from build123d import *

# Parameters (mm, degrees)
SKETCH1_R           = 2.4
BOSS_EXTRUDE1_DEPTH = 5
SKETCH2_R           = 2.4
CUT_EXTRUDE1_DEPTH  = 5
CUT_EXTRUDE2_DEPTH  = 1
SKETCH5_R           = 5
SKETCH5_R_2         = 1
BOSS_EXTRUDE2_DEPTH = 3
SKETCH6_R           = 2
CUT_EXTRUDE3_DEPTH  = 1


with BuildPart() as part:
    # Sketch1 → Boss-Extrude1 (new body)
    with BuildSketch(Plane(origin=(0, 0, 0), x_dir=(0.999757303, -0.022030336, 0), z_dir=(0, 0, 1))):
        with BuildLine():
            Line((-49.372163993, 87.590629426), (-29.904437649, 103.275259833))
            ThreePointArc((-29.904437649, 103.275259833), (-22.873966299, 102.518640646), (-23.630585486, 95.488169295))
            Line((-23.630585486, 95.488169295), (-43.09831183, 79.803538889))
            ThreePointArc((-43.09831183, 79.803538889), (-50.12878318, 80.560158076), (-49.372163993, 87.590629426))
        make_face()
        with Locations((-26.767511567, 99.381714564)):
            Circle(SKETCH1_R, mode=Mode.SUBTRACT)
    extrude(amount=BOSS_EXTRUDE1_DEPTH)

    # Sketch2 → Cut-Extrude1 (cut)
    with BuildSketch(Plane(origin=(0, 0, 0), x_dir=(-1, 0, 0), z_dir=(0, 0, -1))):
        with Locations((44.380141864, 84.695348924)):
            Circle(SKETCH2_R)
    extrude(amount=-CUT_EXTRUDE1_DEPTH, mode=Mode.SUBTRACT)

    # Sketch4 → Cut-Extrude2 (cut)
    with BuildSketch(Plane(origin=(0, 0, 0), x_dir=(-1, 0, 0), z_dir=(0, 0, -1))):
        Polygon((38.237095204, 87.532175923), (40.067328392, 89.909200633), (41.210775583, 87.135659842), align=None)
    extrude(amount=-CUT_EXTRUDE2_DEPTH, mode=Mode.SUBTRACT)

    # Sketch5 → Boss-Extrude2 (add)
    with BuildSketch(Plane.XY.offset(5)):
        with Locations((-24.571602608, 99.947292162)):
            Circle(SKETCH5_R)
        with Locations((-24.571602608, 99.947292162)):
            Circle(SKETCH5_R_2, mode=Mode.SUBTRACT)
    extrude(amount=BOSS_EXTRUDE2_DEPTH)

    # Sketch6 → Cut-Extrude3 (cut)
    with BuildSketch(Plane.XY.offset(8)):
        with Locations((-24.571602608, 99.947292162)):
            Circle(SKETCH6_R)
    extrude(amount=-CUT_EXTRUDE3_DEPTH, mode=Mode.SUBTRACT)


solid = part.part
Build history of the part. All positions in model axes, mm. A direction names the side the tool comes from. Coordinates: 2 decimals unless noted, no trailing zeros. Write each loop counter-clockwise with the first axis right and the second up, starting at its lowest first coordinate (ties: lowest second). Pieces come first, ordered by that corner, then holes. Notation, with made-up numbers: (-25.5, 63) -> (-8.5, 63) arc R15 cw to (-8.5, 78) -> close; hole circle Ø5 at (47.25, 78). An arc over 180 degrees is marked (long way). Use CSV: the item, a comma, the result in double quotes. Start each with the question number.
Q1. Flat gauge pins, fed straight in: pin 1 Ø1.2 at (x, y) = (-24.5, 100.5) entering from +Z; pin 2 Ø1 at (x, y) = (-41.5, 93.5) entering from +Z. Where does each tip first touch, or does it go through?
Q2. 3-axis set-ups, long thin cutter, end or side, ignore diameter. For faces 4 (the cylindrical face through (-24.832, 102.333, 2.465)), 5 (the cylindrical face through (-43.86, 82.352, 2.465)), 6 (the cylindrical face through (-23.496, 101.634, 7.507)): which of +Z, -Z, +X, -X, +Y, -Y reach the whole face in a straight line?
Q3. Cut at C-C, the plane y = 96.5. List the corners of the cut face in (x, z), then the cut area to 3 significant figures.
Q4. Drill centre lines: probe 1 along Z at (x, y) = (-41.25, 91.25); probe 2 along Y at (x, z) = (-24.25, 6.5); probe 3 along X at (y, z) = (86.5, 1). Where is each one in solid material? Low to high.
Q5. Cut at D-D, the plane x = -40.5. List the corners of the cut face in (y, z), then the cut area to 3 significant figures.
Q6. Cut at B-B, the plane z = 3.25. List the corners of the cut face in (x, y), then the cut area to 3 significant figures.
Q7. Pull direction X, two halves, no side cores. Call faces 1 (the flat face through (-22, 100, 8)), 2 (the flat face through (-40.63, 88.54, 0.49)), 3 (the flat face through (-37.66, 96.18, 2.46)): released by +X, released by -X, zero draft, split by the parting line, or undercut.
Q8. Cut at A-A, the plane x = -43.5. List the corners of the cut face in (y, z).
Checked values:
1,pin 1,"stops at z = 7"
1,pin 2,"stops at z = 5"
2,face 4,"-Z"
2,face 5,"+Z, -Z"
2,face 6,"+Z"
3,outline,"(-37.24, 0) -> (-20.95, 0) -> (-20.95, 8) -> (-28.19, 8) -> (-28.19, 5) -> (-37.24, 5) -> close"
3,area,"103 mm²"
4,probe 1,"z = 0 to 5"
4,probe 2,"y = 94.96 to 99, 100.89 to 104.94"
4,probe 3,"x = -49.04 to -45.96, -42.8 to -33.84"
5,outline,"(81.37, 0) -> (87.23, 0) -> (87.23, 1) -> (88.86, 1) -> (88.86, 0) -> (93.99, 0) -> (93.99, 5) -> (81.37, 5) -> close"
5,area,"61.5 mm²"
6,outline,"(-47.43, 88.66) arc R5 ccw to (-41.33, 80.73) -> (-21.52, 95.99) arc R5 ccw to (-27.62, 103.91) -> close; hole circle Ø4.8 at (-44.38, 84.7); hole circle Ø4.8 at (-24.57, 99.95)"
6,area,"292 mm²"
7,face 1,"zero draft"
7,face 2,"undercut"
7,face 3,"released by -X"
8,outline,"(79.77, 0) -> (82.46, 0) -> (82.46, 5) -> (79.77, 5) -> close; (86.93, 0) -> (91.68, 0) -> (91.68, 5) -> (86.93, 5) -> close"
